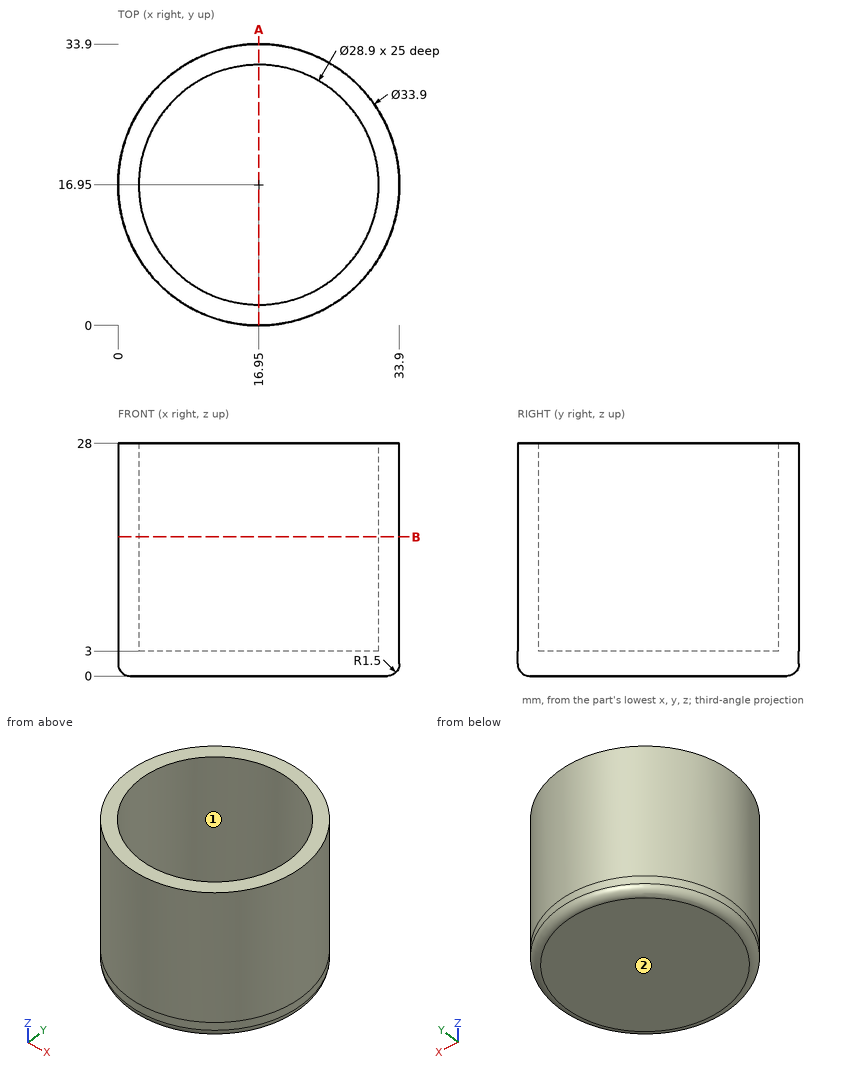
Geometry check sheet. Reference: drawing and pictorial views, mm from the part's lowest x, y, z. Give positions to 0.01 mm unless a question says otherwise; leave off trailing zeros. Order: outer loops, then holes, each group sorted by start corner. A loop starts at its lowest first (then second) coordinate and runs counter-clockwise, first axis right, second up. Notation, with made-up numbers: M -3,50 L 43,50 A19 cw 43,78 Z; hole C -27,-22 d3. An arc over 180 degrees is marked long. Answer in a Markdown table with one row per item. Add a question column.
Q1. Release check for a two-part mould opening along Y. For the marked faces 1 and 2 record: released by +Y, released by -Y, zero draft, split by the parting line, or undercut.
Q2. Gauge pin test, flat ends, axial feed: pin 1 Ø1 at (x, y) = (23, 7.5) entering from +Z; pin 2 Ø6 at (x, z) = (10, 22) entering from +Y; pin 3 Ø2 at (y, z) = (30.5, 9) entering from +X. Record the tip position at first contact, or that the pin passes through.
Q3. Sectioned sample at B-B, the plane z = 16.75. Record the boundary of the cut face in (x, y).
Q4. Thickness scan on L1, parallel to Y at x = 16.95, z = 22; L2, parallel to Z at x = 24, y = 23.5; L3, parallel to Y at x = 22, z = 12. Record the ranges inside material, lowest first.
Q5. Sectioned sample at A-A, the plane x = 16.95. Record the boundary of the cut face in (y, z), and give its area (3 significant figures).
Verdict:
| question | item | result |
|---|---|---|
| 1 | face 1 | undercut |
| 1 | face 2 | zero draft |
| 2 | pin 1 | z = 3 |
| 2 | pin 2 | y = 33.43 |
| 2 | pin 3 | x = 28.34 |
| 3 | outline | C 16.95,16.95 d33.9; hole C 16.95,16.95 d28.9 |
| 4 | L1 | 0 to 2.5, 31.4 to 33.9 |
| 4 | L2 | 0 to 3 |
| 4 | L3 | 0.77 to 3.41, 30.49 to 33.13 |
| 5 | outline | M 0,1.5 A1.5 ccw 1.5,0 L 32.4,0 A1.5 ccw 33.9,1.5 L 33.9,28 L 31.4,28 L 31.4,3 L 2.5,3 L 2.5,28 L 0,28 Z |
| 5 | area | 226 mm² |
